Part model, mm, in its own coordinate system. A direction names the side the tool comes from. Coordinates: 2 decimals unless noted, no trailing zeros. Write each loop counter-clockwise with the first axis right and the second up, starting at its lowest first coordinate (ties: lowest second). Pieces come first, ordered by that corner, then holes. Notation, with made-up numbers: M 9,37 L 52,37 A21 ccw 52,58 Z; hole C 60.25,20.25 d10. An arc over 180 degrees is marked long. Use a Markdown table: item, result. Add a question column.
Q1. Mould opens along Z. For faces 6 (the flat face through (99, 139, 0)), 7 (the flat face through (200, 173, 25)), 8 (the cylindrical face through (45, 145, 110)) say: released by +Z, released by -Z, zero draft, split by the parting line, or undercut.
Q2. Slice it at A-A on z = 110. Write the cut outline in (x, y).
Q3. Slice it at D-D on x = 33. Write the cut outline in (y, z), then the cut area to 3 significant figures.
Q4. Wall check: L1, parallel to Y at x = 65, z = 37.5; L2, parallel to X at y = 138.5, z = 112.5; L3, parallel to Z at x = 44.25, y = 150. Give the ranges that are in metal, low to high. Write a range as from..to.
Q5. Pin check, flat tips, straight feed: pin 1 Ø24 at (y, z) = (152, 111.5) entering from +X; pin 2 Ø2.5 at (x, y) = (65, 0) entering from +Z; pin 3 Ø8 at (x, y) = (101, 178.5) entering from +Z; pin 4 Ø6 at (x, y) = (25.5, 153) entering from +Z. Stop position of each tip, or through.
Q6. Tool access for faces 1 (the flat face through (35, 220, 25)), 2 (the flat face through (30, 130, 77)), 3 (the flat face through (20, 149.7, 104.8)), 4 (the flat face through (32, -32, 45)), 5 (the flat face through (50, 150, 85)): list every direction of +Z, -Z, +X, -X, +Y, -Y with a clear straight run to the whole face (end or side of a thin tool).
Q7. Slice it at C-C on z = 23. Write the cut outline in (x, y), then the cut area to 3 significant figures.
Q8. Slice it at B-B on y = 150. Write the cut outline in (x, z), then the cut area to 3 significant figures.
from build123d import *

# Parameters (mm, degrees)
P_IDAT_VYSUNUT_M1_DEPTH  = 50
SKICA2_W                 = 130
SKICA2_H                 = 5
P_IDAT_VYSUNUT_M2_DEPTH  = 65
SKICA3_W                 = 65
SKICA3_H                 = 65
ODEBRAT_VYSUNUT_M1_DEPTH = 5
SKICA4_W                 = 40
SKICA4_H                 = 40
P_IDAT_VYSUNUT_M3_DEPTH  = 40
SKICA5_W                 = 10
SKICA5_H                 = 40
P_IDAT_VYSUNUT_M4_DEPTH  = 30
SKICA6_R                 = 5
ODEBRAT_VYSUNUT_M2_DEPTH = 40
SKICA7_R                 = 2.5
ODEBRAT_VYSUNUT_M3_DEPTH = 55
SKICA8_R                 = 1.5
ODEBRAT_VYSUNUT_M4_DEPTH = 50


with BuildPart() as part:
    # Skica1 → Přidat vysunutím1 (new body)
    with BuildSketch(Plane.XY):
        Polygon((0, 0), (200, 0), (200, 350), (70, 220), (0, 220), align=None)
    extrude(amount=P_IDAT_VYSUNUT_M1_DEPTH)

    # Skica2 → Přidat vysunutím2 (add)
    with BuildSketch(Plane.XZ):
        with Locations((65, 47.5)):
            Rectangle(SKICA2_W, SKICA2_H)
    extrude(amount=P_IDAT_VYSUNUT_M2_DEPTH)

    # Skica3 → Odebrat vysunutím1 (cut)
    with BuildSketch(Plane.XY.offset(50)):
        with Locations((97.5, -32.5)):
            Rectangle(SKICA3_W, SKICA3_H)
    extrude(amount=-ODEBRAT_VYSUNUT_M1_DEPTH, mode=Mode.SUBTRACT)

    # Skica4 → Přidat vysunutím3 (add)
    with BuildSketch(Plane.XY.offset(50)):
        with Locations((30, 150)):
            Rectangle(SKICA4_W, SKICA4_H)
    extrude(amount=P_IDAT_VYSUNUT_M3_DEPTH)

    # Skica5 → Přidat vysunutím4 (add)
    with BuildSketch(Plane.XY.offset(90)):
        with Locations((15, 150)):
            Rectangle(SKICA5_W, SKICA5_H)
        with Locations((45, 150)):
            Rectangle(SKICA5_W, SKICA5_H)
    extrude(amount=P_IDAT_VYSUNUT_M4_DEPTH)

    # Skica6 → Odebrat vysunutím2 (cut)
    with BuildSketch(Plane(origin=(50, 0, 0), x_dir=(0, 0, -1), z_dir=(1, 0, 0))):
        with Locations(Location((-110, 150, 0), (0, 0, 90))):
            Circle(SKICA6_R)
    extrude(amount=-ODEBRAT_VYSUNUT_M2_DEPTH, mode=Mode.SUBTRACT)

    # Skica7 → Odebrat vysunutím3 (cut)
    with BuildSketch(Plane.XY.offset(50)):
        with Locations((65, 75)):
            Circle(SKICA7_R)
    extrude(amount=-ODEBRAT_VYSUNUT_M3_DEPTH, mode=Mode.SUBTRACT)

    # Skica8 → Odebrat vysunutím4 (cut)
    with BuildSketch(Plane.XY.offset(50)):
        with Locations((65, 0)):
            Circle(SKICA8_R)
    extrude(amount=-ODEBRAT_VYSUNUT_M4_DEPTH, mode=Mode.SUBTRACT)


solid = part.part
Recorded:
| question | item | result |
|---|---|---|
| 1 | face 6 | released by -Z |
| 1 | face 7 | zero draft |
| 1 | face 8 | undercut |
| 2 | outline | M 10,130 L 20,130 L 20,145 L 10,145 Z; M 10,155 L 20,155 L 20,170 L 10,170 Z; M 40,130 L 50,130 L 50,145 L 40,145 Z; M 40,155 L 50,155 L 50,170 L 40,170 Z |
| 3 | outline | M -65,45 L 0,45 L 0,0 L 220,0 L 220,50 L 170,50 L 170,90 L 130,90 L 130,50 L -65,50 Z |
| 3 | area | 12,900 mm² |
| 4 | L1 | 1.5..72.5, 77.5..220 |
| 4 | L2 | 10..20, 40..50 |
| 4 | L3 | 0..105, 115..120 |
| 5 | pin 1 | x = 50 |
| 5 | pin 2 | through |
| 5 | pin 3 | z = 50 |
| 5 | pin 4 | z = 90 |
| 6 | face 1 | +Z, -Z, -X, +Y |
| 6 | face 2 | +Z, +X, -X, -Y |
| 6 | face 3 | +Z, +Y, -Y |
| 6 | face 4 | -Z, +X, -X, -Y |
| 6 | face 5 | +Z, +X, +Y, -Y |
| 7 | outline | M 0,0 L 63.5,0 A1.5 cw 66.5,0 L 200,0 L 200,350 L 70,220 L 0,220 Z; hole C 65,75 d5 |
| 7 | area | 52,400 mm² |
| 8 | outline | M 0,0 L 200,0 L 200,50 L 50,50 L 50,105 L 40,105 L 40,90 L 20,90 L 20,105 L 10,105 L 10,50 L 0,50 Z; M 10,115 L 20,115 L 20,120 L 10,120 Z; M 40,115 L 50,115 L 50,120 L 40,120 Z |
| 8 | area | 12,000 mm² |
